```python
from build123d import *


with BuildPart() as part:
    # Sketch1 → Revolve1 (revolve)
    with BuildSketch(Plane.XY):
        Polygon((0, 6.35), (0, 12.5), (30, 12.5), (30, 20), (33, 25), (35, 25), (35, 32.5), (40, 32.5), (40, 40), (220, 40), (220, 30), (185, 30), (185, 5), (50, 5), (50, 6.35), align=None)
    revolve(axis=Axis((1.424970928, 0, 0), (1, 0, 0)))


solid = part.part
```
Verification items for the finished model (mm, model axes). A direction names the side the tool comes from. Coordinates: 2 decimals unless noted, no trailing zeros. Loops run counter-clockwise (first coordinate to the right, second up) from the corner with the lowest first, then second, coordinate; pieces in that order, holes last. Notation, with made-up numbers: (63, -7.5) -> (81, -7.5) arc R19 cw to (81, 1.5) -> close; hole circle Ø4 at (-27, -2.75). An arc over 180 degrees is marked (long way). Answer in a Markdown table with one row per item.
1) Section check D-D (x = 80.5). Record the cut outline in (y, z).
The answers:
| item | result |
|---|---|
| outline | circle Ø80 at (0, 0); hole circle Ø10 at (0, 0) |
2) Depth check by flat-ended pin: P1, Ø6, axis at y = -18.5, z = 15.5, coming from the +X side; P2, Ø1, axis at x = 104.5, z = -17.5, coming from the +Y side; P3, Ø8, axis at x = 124, y = 10, coming from the -Z side. Enter the tip coordinate at first touch or a pass-through.
The answers:
| item | result |
|---|---|
| P1 | stops at x = 185 |
| P2 | stops at y = 36.21 |
| P3 | stops at z = -39.55 |
3) Access from +Z, -Z, +X, -X, +Y, -Y to the whole of each face (thin tool, end or side, straight path). Record for faces 1 (the face through (34.014, 23.846, 7.509)), 2 (the face through (0, 6, 3)), 3 (the face through (185, 0, -6)).
The answers:
| item | result |
|---|---|
| face 1 | -X |
| face 2 | +Z, -Z, -X, +Y, -Y |
| face 3 | +X |
4) Draft check along Z on faces 4 (the face through (30.2, 19.4, 6.1)), 5 (the face through (50, -2, -5)), 6 (the face through (35, -17, -19)). Enter one of: released by +Z, released by -Z, zero draft, split by the parting line, or undercut.
The answers:
| item | result |
|---|---|
| face 4 | split by the parting line |
| face 5 | undercut |
| face 6 | zero draft |
5) Section check C-C (x = 45.5). Record the cut outline in (y, z).
The answers:
| item | result |
|---|---|
| outline | circle Ø80 at (0, 0); hole circle Ø12.7 at (0, 0) |
6) Scan lines: line 1 along Z through (x, y) = (17.5, 0); line 2 along X through (y, z) = (26.5, -29.5); line 3 along Z through (x, y) = (189.5, 6). Record each from-to range of solid material in increasing order. Write a range as from..to.
The answers:
| item | result |
|---|---|
| line 1 | z = -12.5..-6.35, 6.35..12.5 |
| line 2 | x = 40..220 |
| line 3 | z = -39.55..-29.39, 29.39..39.55 |
